Part model, mm, in its own coordinate system. Give positions to 0.01 mm unless a question says otherwise; leave off trailing zeros. Order: outer loops, then holes, each group sorted by start corner. A loop starts at its lowest first (then second) coordinate and runs counter-clockwise, first axis right, second up.
from build123d import *

# Parameters (mm, degrees)
ESQUISSE1_W        = 19
ESQUISSE1_H        = 70
ESQUISSE1_R        = 2.9
ESQUISSE1_H_2      = 10
ESQUISSE1_W_2      = 21.5
ESQUISSE1_R_2      = 1.3
BOSS_EXTRU_1_DEPTH = 3
CONG_1_R           = 10
CONG_2_R           = 1


with BuildPart() as part:
    # Esquisse1 → Boss.-Extru.1 (new body)
    # profile 1 of 3: a face of its own
    with BuildSketch(Plane.XY.offset(23)):
        with Locations((9.5, 112)):
            Rectangle(ESQUISSE1_W, ESQUISSE1_H)
        with Locations((10, 86)):
            Circle(ESQUISSE1_R, mode=Mode.SUBTRACT)
    # profile 2 of 3: a face of its own
    with BuildSketch(Plane.XY.offset(23)):
        with Locations((9.5, 152)):
            Rectangle(ESQUISSE1_W, ESQUISSE1_H_2)
    # profile 3 of 3: a face of its own
    with BuildSketch(Plane.XY.offset(23)):
        with Locations((29.75, 152)):
            Rectangle(ESQUISSE1_W_2, ESQUISSE1_H_2)
        with Locations((36.5, 153)):
            Circle(ESQUISSE1_R_2, mode=Mode.SUBTRACT)
    extrude(amount=BOSS_EXTRU_1_DEPTH)

    # Congé1
    cong_1_edges = [part.edges().sort_by_distance(p)[0] for p in [
        (0, 157, 24.5),
        (19, 147, 24.5),
    ]]
    fillet(cong_1_edges, radius=CONG_1_R)

    # Congé2
    cong_2_edges = [part.edges().sort_by_distance(p)[0] for p in [
        (25.25, 157, 23),
        (40.5, 152, 23),
        (19, 107, 23),
        (9.5, 77, 23),
        (0, 112, 23),
        (9.5, 77, 26),
        (40.5, 157, 24.5),
        (19, 77, 24.5),
        (0, 77, 24.5),
        (19, 107, 26),
        (34.75, 147, 23),
        (34.75, 147, 26),
        (40.5, 152, 26),
        (2.928932188, 154.071067812, 23),
        (2.928932188, 154.071067812, 26),
        (25.25, 157, 26),
        (21.928932188, 144.071067812, 23),
        (21.928932188, 144.071067812, 26),
        (0, 112, 26),
    ]]
    fillet(cong_2_edges, radius=CONG_2_R)


solid = part.part
Item 1: Drill centre lines: probe 1 along Y at (x, z) = (10, 24.2); probe 2 along Y at (x, z) = (36.5, 23.9); probe 3 along X at (y, z) = (153, 23.6). Where is each one in solid material? Low to high.
Item 2: Drop flat-ended pins along their axis: P1, Ø2.5, axis at x = 36.5, y = 153, coming from the +Z side; P2, Ø0.5, axis at x = 36, z = 24.5, coming from the -Y side; P3, Ø1.1, axis at y = 99, z = 24.5, coming from the +X side. Give the stop position or say it passes through.
Item 3: Band-saw the part on B-B on x = 36.5. List the corners of the cut face in (y, z), plus the area to 3 significant figures.
Item 4: Pull direction X, two halves, no side cores. Call faces 1 (the face through (35.542, 153.879, 24.479)), 2 (the face through (2.85, 153.99, 24.51)), 3 (the face through (11, 118, 26)): released by +X, released by -X, zero draft, split by the parting line, or undercut.
Item 5: Band-saw the part on A-A on y = 86. List the corners of the cut face in (x, z), plus the area to 3 significant figures.
Item 6: Band-saw the part on C-C on x = 31. List the corners of the cut face in (y, z), plus the area to 3 significant figures.
Item 7: Band-saw the part on D-D on y = 103. List the corners of the cut face in (x, z).
Working result:
1. probe 1: y = 77 to 83.1, 88.9 to 157
1. probe 2: y = 147.01 to 151.7, 154.3 to 156.99
1. probe 3: x = 2.1 to 35.2, 37.8 to 40.42
2. P1: passes through
2. P2: stops at y = 147
2. P3: stops at x = 19
3. outline: (147, 24) arc R1 ccw to (148, 23) - (151.7, 23) - (151.7, 26) - (148, 26) arc R1 ccw to (147, 25) - close; (154.3, 23) - (156, 23) arc R1 ccw to (157, 24) - (157, 25) arc R1 ccw to (156, 26) - (154.3, 26) - close
3. area: 21.3 mm2
4. face 1: undercut
4. face 2: released by -X
4. face 3: zero draft
5. outline: (0, 24) arc R1 ccw to (1, 23) - (7.1, 23) - (7.1, 26) - (1, 26) arc R1 ccw to (0, 25) - close; (12.9, 23) - (18, 23) arc R1 ccw to (19, 24) - (19, 25) arc R1 ccw to (18, 26) - (12.9, 26) - close
5. area: 38.7 mm2
6. outline: (147, 24) arc R1 ccw to (148, 23) - (156, 23) arc R1 ccw to (157, 24) - (157, 25) arc R1 ccw to (156, 26) - (148, 26) arc R1 ccw to (147, 25) - close
6. area: 29.1 mm2
7. outline: (0, 24) arc R1 ccw to (1, 23) - (18, 23) arc R1 ccw to (19, 24) - (19, 25) arc R1 ccw to (18, 26) - (1, 26) arc R1 ccw to (0, 25) - close
